Geometry: final body of the model. Coordinates: model frame, mm. Face numbers are marked on the shaded views. A direction names the side the tool comes from. Give positions to 0.01 mm unless a question says otherwise; leave off trailing zeros. Order: outer loops, then holes, each group sorted by start corner. A loop starts at its lowest first (then second) coordinate and runs counter-clockwise, first axis right, second up. Notation, with made-up numbers: (48.5, -18) -> (92.5, -18) arc R20 cw to (92.5, -3) -> close; hole circle Ø3 at (61, 26). An arc over 180 degrees is marked (long way). Write item = value, one per line.
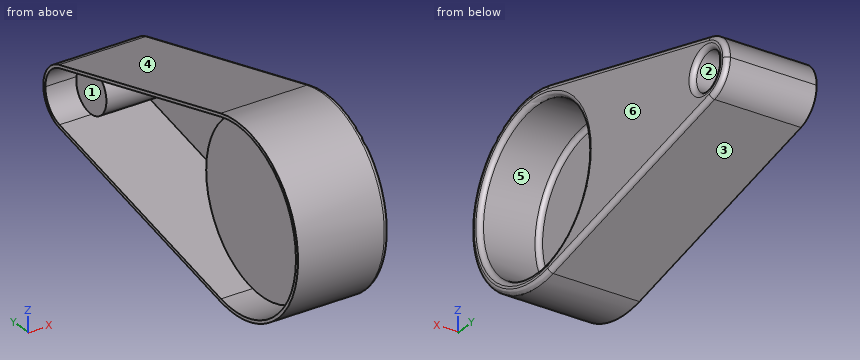
```python
from build123d import *

# Parameters (mm, degrees)
F1_DEPTH = 76.2
F2_R     = 66.675
F2_R_2   = 15.875
F3_DEPTH = 50.8
F4_T     = -2.54
F5_R     = 3.81
F6_R     = 3.81


with BuildPart() as f1:
    # F0 (on Right) → F1 (new body)
    with BuildSketch(Plane.YZ):
        with BuildLine():
            ThreePointArc((18.4812146278, -73.9248585111), (60.0612543768, -46.8944103565), (76.2, 0))
            ThreePointArc((76.2, 0), (60.0612543768, 46.8944103565), (18.4812146278, 73.9248585111))
            ThreePointArc((18.4812146278, 73.9248585111), (-76.2, 0), (18.4812146278, -73.9248585111))
        make_face()
        with BuildLine():
            ThreePointArc((18.4812146278, 73.9248585111), (60.0612543768, 46.8944103565), (76.2, 0))
            ThreePointArc((76.2, 0), (60.0612543768, -46.8944103565), (18.4812146278, -73.9248585111))
            Line((18.4812146278, -73.9248585111), (215.6141706573, -24.6416195037))
            ThreePointArc((215.6141706573, -24.6416195037), (184.2029995957, -2.7493284703), (210.1666790363, 25.3899931999))
            ThreePointArc((210.1666790363, 25.3899931999), (212.910735745, 25.1636515369), (215.6141706573, 24.6416195037))
            Line((215.6141706573, 24.6416195037), (18.4812146278, 73.9248585111))
        make_face()
        with BuildLine():
            Line((210.1666790363, 25.3899931999), (215.6141706573, 24.6416195037))
            ThreePointArc((215.6141706573, 24.6416195037), (212.910735745, 25.1636515369), (210.1666790363, 25.3899931999))
        make_face()
        with BuildLine():
            ThreePointArc((234.8537657814, 0), (229.474183907, 15.6314701188), (215.6141706573, 24.6416195037))
            Line((215.6141706573, 24.6416195037), (210.1666790363, 25.3899931999))
            ThreePointArc((210.1666790363, 25.3899931999), (184.2029995957, -2.7493284703), (215.6141706573, -24.6416195037))
            ThreePointArc((215.6141706573, -24.6416195037), (229.474183907, -15.6314701188), (234.8537657814, 0))
        make_face()
    extrude(amount=F1_DEPTH)

    # F2 (on face) → F3 (cut)
    with BuildSketch(Plane.YZ.offset(76.2)):
        Circle(F2_R)
        with Locations((209.4537657814, 0)):
            Circle(F2_R_2)
    extrude(amount=-F3_DEPTH, mode=Mode.SUBTRACT)

    # F4
    f4_openings = [f1.faces().sort_by_distance(p)[0] for p in [
        (0, 57.51924, 0),
    ]]
    offset(amount=F4_T, openings=f4_openings, kind=Kind.INTERSECTION)

    # F5
    f5_edges = [f1.edges().sort_by_distance(p)[0] for p in [
        (76.2, -76.2, 0),
        (76.2, 117.047693, 49.283239),
        (76.2, 117.047693, -49.283239),
        (76.2, 234.853766, 0),
        (76.2, -66.675, 0),
        (76.2, 193.578766, 0),
    ]]
    fillet(f5_edges, radius=F5_R)

    # F6
    f6_edges = [f1.edges().sort_by_distance(p)[0] for p in [
        (25.4, -66.675, 0),
        (25.4, 193.578766, 0),
    ]]
    fillet(f6_edges, radius=F6_R)


solid = f1.part
```
1) Reachability of the marked faces 1, 2 and 3 from +Z, -Z, +X, -X, +Y, -Y: full face, straight path, thin tool, end or side. Return the list, or none.
Check sheet entries:
face_1 = -X
face_2 = +X
face_3 = -Z, +X, -X, +Y
2) Mould query, pull axis Z, two halves, no side actions, for the marked faces 4, 5 and 6. Classes: +Z half, -Z half, draft (parallel to the pull), parting line (faces both ways), or undercut.
Check sheet entries:
face_4 = +Z half
face_5 = undercut
face_6 = draft
3) Line query: line 1 (Z direction, x = 53.5, y = 0) (3 decimals); line 2 (Z direction, x = 20, y = 0); line 3 (Z direction, x = 61, y = 193). Output: solid intervals per line, ascending. Write a range as from..to.
Check sheet entries:
line_1 = -76.2..-73.66, -69.215..-66.675, 66.675..69.215, 73.66..76.2
line_2 = -76.2..-73.66, 73.66..76.2
line_3 = -30.3..-27.68, -8.27..8.27, 27.68..30.3
4) Section query A-A (x = 63). Output: boundary loops of the cut face in (y, z) (3 decimals), plus the area to 3 significant figures.
Check sheet entries:
outline = circle Ø138.43 at (0, 0); (18.481, -73.925) -> (215.614, -24.642) arc R25.4 ccw to (215.614, 24.642) -> (18.481, 73.925) arc R76.2 ccw (long way) to start; circle Ø36.83 at (209.454, 0); hole circle Ø133.35 at (0, 0); hole (17.865, -71.461) -> (214.998, -22.177) arc R22.86 ccw to (214.998, 22.177) -> (17.865, 71.461) arc R73.66 ccw (long way) to start; hole circle Ø31.75 at (209.454, 0)
area = 3,240 mm²
5) First-contact query: P1, Ø1, axis at y = -9, z = 60.5, coming from the -X side; P2, Ø6, axis at x = 53.5, y = 83.5, coming from the +Z side; P3, Ø5, axis at x = 29, y = 63, coming from the +Z side. Flat tips, straight axial feed; report the tip coordinate or a pass-through.
Check sheet entries:
P1 = 22.86
P2 = 58.42
P3 = 63.42
